Drawing for the job (mm, zero at the part's lowest x, y, z). A direction names the side the tool comes from. Round coordinates to 2 decimals unless told otherwise and drop trailing zeros. Write each loop counter-clockwise with the first axis right and the second up, starting at its lowest first coordinate (ties: lowest second). Pieces come first, ordered by that corner, then holes. Notation, with made-up numbers: (67.25, -8) - (73.25, -8) arc R13 cw to (73.25, 14) - close; hole circle Ø6 at (43, 79.5). An arc over 180 degrees is marked (long way). One line per question, with ' | ' between items.
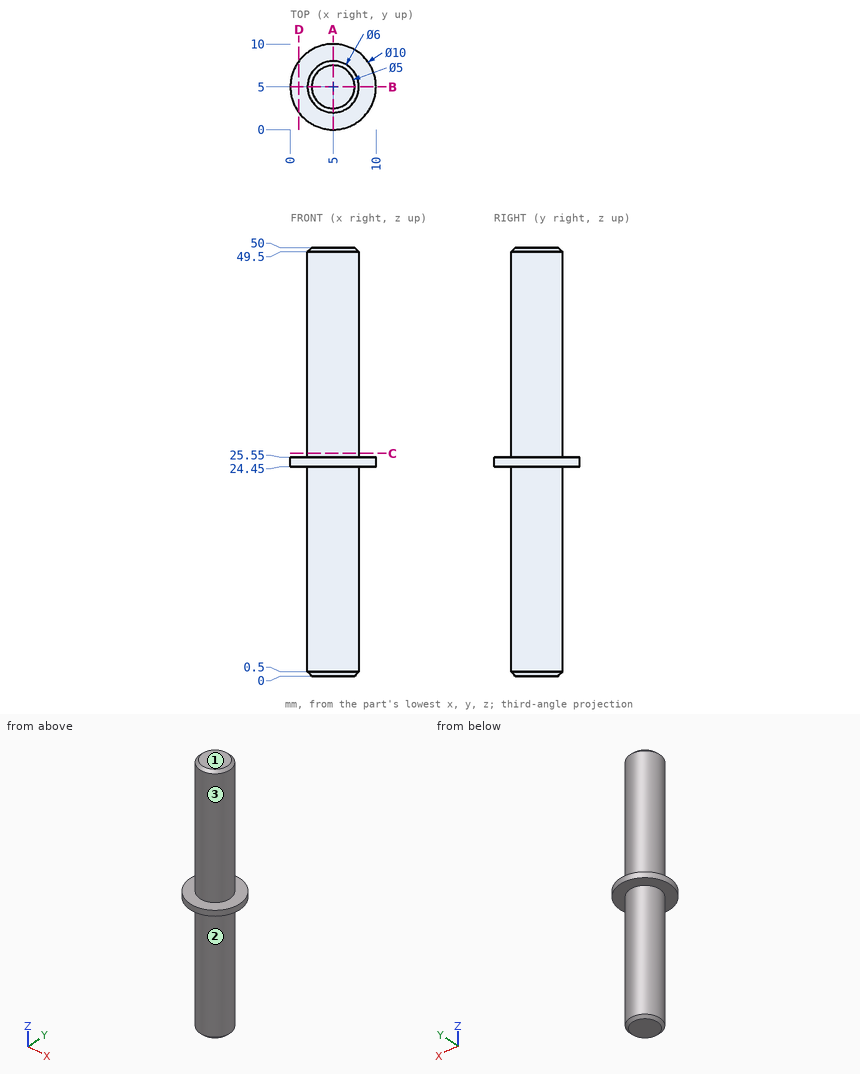
Q1. Drill centre lines: L1, parallel to Z at x = 5, y = 0.5; L2, parallel to X at y = 5.75, z = 45; L3, parallel to X at y = 4.75, z = 3.5. Where is each one in solid material? Low to high. Write a range as from..to.
Found:
L1: 24.45..25.55 | L2: 2.1..7.9 | L3: 2.01..7.99
Q2. Which spindle directions (+Z, -Z, +X, -X, +Y, -Y) get a long thin tool onto all of the face, cutting with end or side? Do the marked faces 1, 2 and 3. Say none if no direction does.
Found:
face 1: +Z, +X, -X, +Y, -Y | face 2: -Z | face 3: +Z
Q3. Saw through at D-D, the plane x = 1. List the corners of the cut face in (y, z), then the cut area to 3 significant figures.
Found:
outline: (2, 24.45) - (8, 24.45) - (8, 25.55) - (2, 25.55) - close | area: 6.60 mm^2
Q4. Saw through at C-C, the plane z = 26. List the corners of the cut face in (x, y).
Found:
outline: circle Ø6 at (5, 5)
Q5. Saw through at A-A, the plane x = 5. List the corners of the cut face in (y, z), then the cut area to 3 significant figures.
Found:
outline: (0, 24.45) - (2, 24.45) - (2, 0.5) - (2.5, 0) - (7.5, 0) - (8, 0.5) - (8, 24.45) - (10, 24.45) - (10, 25.55) - (8, 25.55) - (8, 49.5) - (7.5, 50) - (2.5, 50) - (2, 49.5) - (2, 25.55) - (0, 25.55) - close | area: 304 mm^2
Q6. Drop a flat-ended pin along its axis: pin 1 (3 mm diameter, centred on x = 5, z = 42, fed in from -Y). Give the stop position or say it passes through.
Found:
pin 1: y = 2
